For this review, take the finished solid that the model builds, in its own axes (mm). Face numbers are marked on the shaded views. A direction names the side the tool comes from. Coordinates: 2 decimals unless noted, no trailing zeros. Loops run counter-clockwise (first coordinate to the right, second up) from the corner with the lowest first, then second, coordinate; pieces in that order, holes last. Notation, with made-up numbers: M 19.25,-30 L 76.25,-30 A31 ccw 76.25,-1 Z; hole C -14,51 d9. An arc over 180 degrees is marked long. Answer as a JSON object with one key per item and string values. Group by question number.
Item 1: Tool access review of the marked faces 1 and 2: name each direction out of +Z, -Z, +X, -X, +Y, -Y from which nothing blocks a thin tool from reaching the whole face with its end or side.
Item 2: Add section B-B (x = 6). State the section outline as (y, z) points.
Item 3: Wall thickness on L1, parallel to X at y = 43, z = 54; L2, parallel to Z at x = 13.5, y = 46; L3, parallel to Y at x = 28, z = 25: over which ranges is each line inside the solid? List them lowest first. Write a range as from..to.
Item 4: Insertion check: pin 1 (8 mm diameter, centred on x = 35, y = 44.5, fed in from +Z); pin 2 (18.5 mm diameter, centred on x = 22, z = 49.5, fed in from -Y); pin 3 (5 mm diameter, centred on x = 17.5, y = 42, fed in from +Z); pin 4 (13.5 mm diameter, centred on y = 55.5, z = 46.5, fed in from +X). Each pin has a flat end and moves straight along its axis. Give the tip position at first contact, or say it passes through.
Item 5: Add section D-D (z = 24.5). State the section outline as (x, y) points, then the cut area to 3 significant figures.
Item 6: Add section A-A (z = 48). State the section outline as (x, y) points, then the cut area to 3 significant figures.
Item 7: Add section C-C (y = 52.5). State the section outline as (x, z) points.
from build123d import *

# Parameters (mm, degrees)
BOSS_EXTRUDE1_DEPTH = 40
CUT_EXTRUDE1_REACH  = 143.085
SKETCH2_R           = 5
CUT_EXTRUDE2_REACH  = 138.298
SKETCH3_W           = 16
SKETCH3_H           = 33
SKETCH4_W           = 16
SKETCH4_H           = 32
CUT_EXTRUDE4_DEPTH  = 40


with BuildPart() as part:
    # Sketch1 → Boss-Extrude1 (new body)
    with BuildSketch(Plane(origin=(0, 0, 0), x_dir=(0, 0, -1), z_dir=(1, 0, 0))):
        Polygon((-102.239092363, 74.801270189), (-107.239092363, 66.141016151), (-59.019237886, 38.301270189), (-22.113248654, 38.301270189), (0, 0), (8.660254038, 5), (-16.339745962, 48.301270189), (-56.339745962, 48.301270189), align=None)
    extrude(amount=BOSS_EXTRUDE1_DEPTH)

    # Sketch2 → Cut-Extrude1 (cut, up to next)
    with BuildSketch(Plane(origin=(0, 5, -8.660254038), x_dir=(-1, 0, 0), z_dir=(0, 0.4999999999999983, -0.8660254037844396)), mode=Mode.PRIVATE) as cut_extrude1_sk1:
        with Locations(Location((-20, 35, 0), (0, 0, 90))):
            Circle(SKETCH2_R)
    cut_extrude1_tool1 = extrude(cut_extrude1_sk1.sketch, amount=-CUT_EXTRUDE1_REACH, mode=Mode.PRIVATE) & part.part
    # Sketch2 → Cut-Extrude1 (cut, up to next)
    with BuildSketch(Plane(origin=(0, 5, -8.660254038), x_dir=(-1, 0, 0), z_dir=(0, 0.4999999999999983, -0.8660254037844396)), mode=Mode.PRIVATE) as cut_extrude1_sk2:
        with Locations(Location((-20, 15, 0), (0, 0, 90))):
            Circle(SKETCH2_R)
    cut_extrude1_tool2 = extrude(cut_extrude1_sk2.sketch, amount=-CUT_EXTRUDE1_REACH, mode=Mode.PRIVATE) & part.part
    add(cut_extrude1_tool1.solids().sort_by_distance((20, 35.310889, 8.839746))[0], mode=Mode.SUBTRACT)
    add(cut_extrude1_tool2.solids().sort_by_distance((20, 17.990381, -1.160254))[0], mode=Mode.SUBTRACT)

    # Sketch3 → Cut-Extrude2 (cut, up to next)
    with BuildSketch(Plane(origin=(0, 11.830127019, -6.830127019), x_dir=(1, 0, 0), z_dir=(0, 0.8660254037844383, -0.5000000000000009)), mode=Mode.PRIVATE) as cut_extrude2_sk1:
        with Locations((20, -89.442286341)):
            Rectangle(SKETCH3_W, SKETCH3_H)
    cut_extrude2_tool1 = extrude(cut_extrude2_sk1.sketch, amount=-CUT_EXTRUDE2_REACH, mode=Mode.PRIVATE) & part.part
    add(cut_extrude2_tool1.solids().sort_by_distance((20, 56.55127, 70.629165))[0], mode=Mode.SUBTRACT)

    # Sketch4 → Cut-Extrude4 (cut)
    with BuildSketch(Plane(origin=(0, 48.301270189, 0), x_dir=(1, 0, 0), z_dir=(0, 1, 0))):
        with Locations((20, -45.339745962)):
            Rectangle(SKETCH4_W, SKETCH4_H)
    extrude(amount=-CUT_EXTRUDE4_DEPTH, mode=Mode.SUBTRACT)


solid = part.part
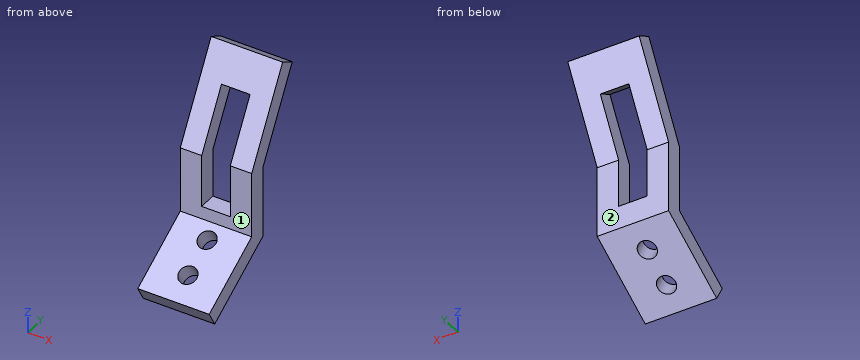
From the geometry:
{
 "1": {"face 1": "+Z, +X, -X, -Y", "face 2": "-Z, +X, -X, +Y"},
 "2": {"outline": "M 0,0 L 5,-8.66 L 48.3,16.34 L 48.3,56.34 L 74.8,102.24 L 66.14,107.24 L 38.3,59.02 L 38.3,22.11 Z"},
 "3": {"L1": "x = 0..12, 28..40", "L2": "z = 15.01..29.34", "L3": "y = 38.3..48.3"},
 "4": {"pin 1": "stops at z = 76.68", "pin 2": "stops at y = 38.3", "pin 3": "stops at z = 29.34", "pin 4": "passes through"},
 "5": {"outline": "M 0,38.3 L 40,38.3 L 40,48.3 L 0,48.3 Z", "area": "400 mm²"},
 "6": {"outline": "M 0,38.3 L 12,38.3 L 12,48.3 L 0,48.3 Z; M 28,38.3 L 40,38.3 L 40,48.3 L 28,48.3 Z", "area": "240 mm²"},
 "7": {"outline": "M 0,63.61 L 12,63.61 L 12,83.61 L 0,83.61 Z; M 28,63.61 L 40,63.61 L 40,83.61 L 28,83.61 Z"}
}
